```python
from build123d import *

# Parameters (mm, degrees)
EXTRUDE_1_DEPTH     = 2.4
EXTRUDE_START       = -2.4
SKETCH_2_R          = 2.65
EXTRUDE_2_DEPTH     = 3.9
FILLET_1_R          = 0.5
FILLET_2_R          = 0.1
SKETCH_3_R          = 1.5
CUT_EXTRUDE_1_DEPTH = 6.723453712


with BuildPart() as part:
    # 草图1 → 凸台-拉伸1 (new body)
    with BuildSketch(Plane.XY):
        Polygon((3.175426481, 0), (1.58771324, 2.75), (-1.58771324, 2.75), (-3.175426481, 0), (-1.58771324, -2.75), (1.58771324, -2.75), align=None)
    extrude(amount=EXTRUDE_1_DEPTH)

    # 草图2 → 凸台-拉伸2 (add)
    with BuildSketch(Plane.XY.offset(2.4).offset(EXTRUDE_START)):
        Circle(SKETCH_2_R)
    extrude(amount=EXTRUDE_2_DEPTH)

    # 圆角1
    fillet_1_edges = [part.edges().sort_by_distance(p)[0] for p in [
        (-2.65, 0, 3.9),
    ]]
    fillet(fillet_1_edges, radius=FILLET_1_R)

    # 圆角2
    fillet_2_edges = [part.edges().sort_by_distance(p)[0] for p in [
        (0, 2.75, 2.4),
        (1.58771324, -2.75, 1.2),
        (-1.58771324, -2.75, 1.2),
        (-3.175426481, 0, 1.2),
        (-1.58771324, 2.75, 1.2),
        (1.58771324, 2.75, 1.2),
        (3.175426481, 0, 1.2),
        (-2.38156986, 1.375, 2.4),
        (-2.38156986, -1.375, 2.4),
        (0, -2.75, 2.4),
        (2.38156986, -1.375, 2.4),
        (0, -2.75, 0),
        (-2.38156986, -1.375, 0),
        (-2.38156986, 1.375, 0),
        (2.38156986, 1.375, 2.4),
        (0, 2.75, 0),
        (2.38156986, 1.375, 0),
        (2.38156986, -1.375, 0),
    ]]
    fillet(fillet_2_edges, radius=FILLET_2_R - 0.0001)  # a hair under: the kernel refuses the full size

    # 草图3 → 切除-拉伸1 (cut, through all)
    with BuildSketch(Plane.XY.offset(3.9)):
        Circle(SKETCH_3_R)
    extrude(amount=-CUT_EXTRUDE_1_DEPTH, mode=Mode.SUBTRACT)


solid = part.part
```
Input: part model. Units: mm. Frame: model coordinates. A direction names the side the tool comes from. Give positions to 0.01 mm unless a question says otherwise; leave off trailing zeros. Loops run counter-clockwise (first coordinate to the right, second up) from the corner with the lowest first, then second, coordinate; pieces in that order, holes last. Notation, with made-up numbers: M -8,78.25 L 44,78.25 A23 ccw 44,101.25 Z; hole C 18.5,85.5 d8. An arc over 180 degrees is marked long. Answer as CSV lines item,"result". Start each with the question number.
1. Pin query (flat end, axial travel): P1, Ø2, axis at y = -2, z = 2, coming from the -X side. Return the tip coordinate at first contact, or that it passes through.
2. Reachability of faces 1 (the face through (2.45, -1.01, 2.89)), 2 (the face through (-2.371, 1.394, 1.185)) from +Z, -Z, +X, -X, +Y, -Y: full face, straight path, thin tool, end or side. Return the list, or none.
3. Section C-C on z = 2.55. Return loops of the section in (x, y).
4. Line query: L1, parallel to X at y = 0.05, z = 2.15; L2, parallel to Y at x = 0, z = 1.05; L3, parallel to Y at x = 0, z = 2.75. Output: solid intervals per line, ascending.
5. Section B-B on z = 1.95. Return loops of the section in (x, y), plus the area to 3 significant figures.
Computed values:
1,P1,"stops at x = -2.6"
2,face 1,"+Z"
2,face 2,"+Z, -Z, -X, +Y"
3,outline,"C 0,0 d5.3; hole C 0,0 d3"
4,L1,"x = -3.15 to -1.5, 1.5 to 3.15"
4,L2,"y = -2.75 to -1.5, 1.5 to 2.75"
4,L3,"y = -2.65 to -1.5, 1.5 to 2.65"
5,outline,"M -3.15,-0.05 L -1.62,-2.7 A0.1 ccw -1.53,-2.75 L 1.53,-2.75 A0.1 ccw 1.62,-2.7 L 3.15,-0.05 A0.1 ccw 3.15,0.05 L 1.62,2.7 A0.1 ccw 1.53,2.75 L -1.53,2.75 A0.1 ccw -1.62,2.7 L -3.15,0.05 A0.1 ccw Z; hole C 0,0 d3"
5,area,"19.1 mm²"
